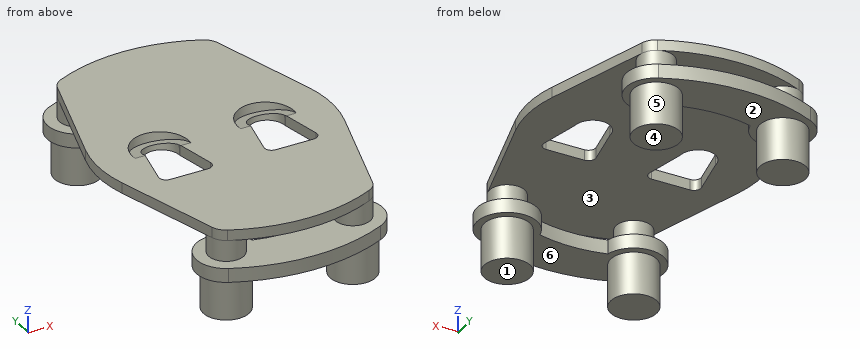
```python
from build123d import *

# Parameters (mm, degrees)
BOSS_EXTRUDE1_DEPTH     = 20
BOSS_EXTRUDE1_2_DEPTH   = 20
SKETCH2_R               = 25
BOSS_EXTRUDE2_DEPTH     = 30
BOSS_EXTRUDE3_DEPTH     = 15
CUT_EXTRUDE1_DEPTH      = 40
CUT_EXTRUDE1_DEPTH_BACK = 51
SKETCH4_R               = 25
SKETCH5_R               = 40
CUT_EXTRUDE2_DEPTH      = 27
SKETCH6_R               = 32.5
BOSS_EXTRUDE4_DEPTH     = 60


with BuildPart() as part:
    # Sketch1 → Boss-Extrude1 (new body)
    with BuildSketch(Plane.XY):
        with BuildLine():
            ThreePointArc((-108.214285714, -1031.864254516), (-116.246402213, -1103.690520511), (-48.376068528, -1078.848113469))
            ThreePointArc((-48.376068528, -1078.848113469), (0, -1072.5), (48.376068528, -1078.848113469))
            ThreePointArc((48.376068528, -1078.848113469), (116.246402213, -1103.690520511), (108.214285714, -1031.864254516))
            ThreePointArc((108.214285714, -1031.864254516), (0, -1007.5), (-108.214285714, -1031.864254516))
        make_face()
    extrude(amount=BOSS_EXTRUDE1_DEPTH)



with BuildPart() as body_2:
    # Sketch1 → Boss-Extrude1 2 (new body)
    with BuildSketch(Plane.XY):
        with BuildLine():
            ThreePointArc((108.214285714, -1488.135745484), (116.246402213, -1416.309479489), (48.376068528, -1441.151886531))
            ThreePointArc((48.376068528, -1441.151886531), (0, -1447.5), (-48.376068528, -1441.151886531))
            ThreePointArc((-48.376068528, -1441.151886531), (-116.246402213, -1416.309479489), (-108.214285714, -1488.135745484))
            ThreePointArc((-108.214285714, -1488.135745484), (0, -1512.5), (108.214285714, -1488.135745484))
        make_face()
    extrude(amount=BOSS_EXTRUDE1_2_DEPTH)


with BuildPart() as part_1:
    add(part.part)

    add(body_2.part)  # Boss-Extrude2 merges body 2
    # Sketch2 → Boss-Extrude2 (add)
    with BuildSketch(Plane.XY.offset(20)):
        with Locations((90, -1070.26334039)):
            Circle(SKETCH2_R)
        with Locations(Location((-90, -1070.26334039, 0), (0, 0, 180))):
            Circle(SKETCH2_R)
        with Locations((-90, -1449.73665961)):
            Circle(SKETCH2_R)
        with Locations(Location((90, -1449.73665961, 0), (0, 0, 180))):
            Circle(SKETCH2_R)
    extrude(amount=BOSS_EXTRUDE2_DEPTH)

    # Sketch3 → Boss-Extrude3 (add)
    with BuildSketch(Plane.XY.offset(50)):
        with BuildLine():
            Line((-113.978732885, -1063.190832404), (-158.259637044, -1213.321447293))
            ThreePointArc((-158.259637044, -1213.321447293), (-165, -1260), (-158.259637044, -1306.678552707))
            Line((-158.259637044, -1306.678552707), (-113.978732885, -1456.809167596))
            ThreePointArc((-113.978732885, -1456.809167596), (-109.002148875, -1465.982223255), (-100.714285714, -1472.324357183))
            ThreePointArc((-100.714285714, -1472.324357183), (0, -1495), (100.714285714, -1472.324357183))
            ThreePointArc((100.714285714, -1472.324357183), (109.002148875, -1465.982223255), (113.978732885, -1456.809167596))
            Line((113.978732885, -1456.809167596), (158.259637044, -1306.678552707))
            ThreePointArc((158.259637044, -1306.678552707), (165, -1260), (158.259637044, -1213.321447293))
            Line((158.259637044, -1213.321447293), (113.978732885, -1063.190832404))
            ThreePointArc((113.978732885, -1063.190832404), (109.002148875, -1054.017776745), (100.714285714, -1047.675642817))
            ThreePointArc((100.714285714, -1047.675642817), (0, -1025), (-100.714285714, -1047.675642817))
            ThreePointArc((-100.714285714, -1047.675642817), (-109.002148875, -1054.017776745), (-113.978732885, -1063.190832404))
        make_face()
        with BuildLine():
            Line((-100, -1260), (-111.986322799, -1316.391215143))
            ThreePointArc((-111.986322799, -1316.391215143), (-109.976306406, -1324.763535962), (-102.204846792, -1328.470332051))
            Line((-102.204846792, -1328.470332051), (-47.795153208, -1328.470332051))
            ThreePointArc((-47.795153208, -1328.470332051), (-40.023693594, -1324.763535962), (-38.013677201, -1316.391215143))
            Line((-38.013677201, -1316.391215143), (-50, -1260))
            ThreePointArc((-50, -1260), (-75, -1235), (-100, -1260))
        make_face(mode=Mode.SUBTRACT)
        with BuildLine():
            Line((100, -1260), (111.986322799, -1316.391215143))
            ThreePointArc((111.986322799, -1316.391215143), (109.976306406, -1324.763535962), (102.204846792, -1328.470332051))
            Line((102.204846792, -1328.470332051), (47.795153208, -1328.470332051))
            ThreePointArc((47.795153208, -1328.470332051), (40.023693594, -1324.763535962), (38.013677201, -1316.391215143))
            Line((38.013677201, -1316.391215143), (50, -1260))
            ThreePointArc((50, -1260), (75, -1235), (100, -1260))
        make_face(mode=Mode.SUBTRACT)
    extrude(amount=BOSS_EXTRUDE3_DEPTH)

    # Sketch4 → Cut-Extrude1 (cut, two sides: drawn at the far end of the back side and taken through both)
    with BuildSketch(Plane(origin=(0, -66.479313163, -248.104174377), x_dir=(-1, 0, 0), z_dir=(0, 0.25881904510252135, 0.9659258262890681)).offset(-CUT_EXTRUDE1_DEPTH_BACK)):
        with Locations((-75, 1230.027041119)):
            Circle(SKETCH4_R)
        with Locations((75, 1230.027041119)):
            Circle(SKETCH4_R)
    extrude(amount=CUT_EXTRUDE1_DEPTH + CUT_EXTRUDE1_DEPTH_BACK, mode=Mode.SUBTRACT)

    # Sketch5 → Cut-Extrude2 (cut)
    with BuildSketch(Plane(origin=(0, -61.302932261, -228.785657851), x_dir=(-1, 0, 0), z_dir=(0, 0.25881904510252135, 0.9659258262890681))):
        with Locations((-75, 1230.027041119)):
            Circle(SKETCH5_R)
        with Locations((75, 1230.027041119)):
            Circle(SKETCH5_R)
    extrude(amount=-CUT_EXTRUDE2_DEPTH, mode=Mode.SUBTRACT)

    # Sketch6 → Boss-Extrude4 (add)
    with BuildSketch(Plane(origin=(0, 0, 0), x_dir=(-1, 0, 0), z_dir=(0, 0, -1))):
        with Locations(Location((90, -1070.26334039, 0), (0, 0, 180))):
            Circle(SKETCH6_R)
        with Locations(Location((-90, -1070.26334039, 0), (0, 0, 180))):
            Circle(SKETCH6_R)
        with Locations(Location((-90, -1449.73665961, 0), (0, 0, 180))):
            Circle(SKETCH6_R)
        with Locations(Location((90, -1449.73665961, 0), (0, 0, 180))):
            Circle(SKETCH6_R)
    extrude(amount=BOSS_EXTRUDE4_DEPTH)


solid = part_1.part
```
Input: part model. Units: mm. Frame: model coordinates. Face numbers are marked on the shaded views. A direction names the side the tool comes from. Give positions to 0.01 mm unless a question says otherwise; leave off trailing zeros. Loops run counter-clockwise (first coordinate to the right, second up) from the corner with the lowest first, then second, coordinate; pieces in that order, holes last.
1) Section query B-B on x = -8.5. Return the cut outline in (y, z), and give its area (3 significant figures).
A:
outline: (-1512.36, 0) - (-1447.31, 0) - (-1447.31, 20) - (-1512.36, 20) - close; (-1494.85, 50) - (-1025.15, 50) - (-1025.15, 65) - (-1494.85, 65) - close; (-1072.69, 0) - (-1007.64, 0) - (-1007.64, 20) - (-1072.69, 20) - close
area: 9,650 mm2
2) Reachability of the marked faces 1, 2 and 3 from +Z, -Z, +X, -X, +Y, -Y: full face, straight path, thin tool, end or side. Return the list, or none.
A:
face 1: -Z, +X, -X, +Y, -Y
face 2: -Z
face 3: none
3) Contact query for flat-ended pins moving along their axis: pin 1 (1 mm diameter, centred on x = 109, y = -1343.5, fed in from -Z); pin 2 (16.5 mm diameter, centred on x = -68, z = 61, fed in from +Y); pin 3 (1.5 mm diameter, centred on x = 61, z = -41.5, fed in from +Y). Output: stop coordinate, or through.
A:
pin 1: stops at z = 50
pin 2: stops at y = -1032.72
pin 3: stops at y = -1054.2
4) Line query: L1, parallel to Z at x = 34.5, y = -1450.5; L2, parallel to Z at x = -91.5, y = -1113.5; L3, parallel to X at y = -1453.5, z = -25. Output: solid intervals per line, ascending.
A:
L1: z = 0 to 20, 50 to 65
L2: z = 50 to 65
L3: x = -122.28 to -57.72, 57.72 to 122.28
5) Section query C-C on y = -1270. Return the cut outline in (x, z), and give its area (3 significant figures).
A:
outline: (-164.7, 50) - (-102.13, 50) - (-102.13, 65) - (-164.7, 65) - close; (-47.87, 50) - (47.87, 50) - (47.87, 65) - (-47.87, 65) - close; (102.13, 50) - (164.7, 50) - (164.7, 65) - (102.13, 65) - close
area: 3,310 mm2
6) Mould query, pull axis X, two halves, no side actions, for the marked faces 4, 5 and 6. Classes: released by +X, released by -X, zero draft, split by the parting line, or undercut.
A:
face 4: zero draft
face 5: undercut
face 6: undercut
7) Section query A-A on z = 12. Return the cut outline in (x, y).
A:
outline: (-108.21, -1488.14) arc R252.5 ccw to (108.21, -1488.14) arc R42.5 ccw (long way) to (48.38, -1441.15) arc R187.5 cw to (-48.38, -1441.15) arc R42.5 ccw (long way) to start; (-108.21, -1031.86) arc R42.5 ccw (long way) to (-48.38, -1078.85) arc R187.5 cw to (48.38, -1078.85) arc R42.5 ccw (long way) to (108.21, -1031.86) arc R252.5 ccw to start
